The model under review builds one solid part; all positions refer to its coordinate system, in mm. A direction names the side the tool comes from. Round coordinates to 2 decimals unless told otherwise and drop trailing zeros. Order: outer loops, then holes, each group sorted by start corner. A loop starts at its lowest first (then second) coordinate and runs counter-clockwise, first axis right, second up. Notation, with made-up numbers: M -15,-19 L 8,-19 A17 ccw 8,-2 Z; hole C -19,73.5 d5. An arc over 180 degrees is marked long. Use a Markdown table: item, result. Add a question column.
1. To check wall thickness, follow probe 1 along X at (y, z) = (-1, 2.85); probe 2 along Y at (x, z) = (-32, 1.4); probe 3 along Y at (x, z) = (-71.5, 2). State the ranges of each line that lie inside material, in increasing order.
2. For faces 1 (the flat face through (-59.466, 21.267, 1.521)), 2 (the flat face through (-34.34, 12.98, 1.52)), 3 (the flat face through (-17, 0, 1)), 4 (the flat face through (-65.527, -1, 2)), list the 3-axis set-ups (+Z, -Z, +X, -X, +Y, -Y) from which the entire face can be reached by the end or side of a thin tool; tool diameter is ignored.
3. Consider section B-B on x = -8.5. State the section outline as (y, z) points.
4. Consider section A-A on z = 2.55. State the section outline as (x, y) points.
5. Insertion check: P1, Ø1, axis at x = -26, z = 0.5, coming from the +Y side; P2, Ø0.9, axis at x = -10.5, z = 2, coming from the -Y side. Each pin has a flat end and moves straight along its axis. Give the tip position at first contact, or say it passes through.
6. Consider section C-C on y = 13.5. State the section outline as (x, z) points, then the cut area to 3 significant figures.
from build123d import *

# Parameters (mm, degrees)
BOSS_EXTRUDE1_DEPTH = 3
BOSS_EXTRUDE2_DEPTH = 3


with BuildPart() as part:
    # Sketch1 → Boss-Extrude1 (new body)
    with BuildSketch(Plane.XY):
        Polygon((0, 0), (-89, 0), (-80.347524158, 26.629582456), align=None)
    extrude(amount=BOSS_EXTRUDE1_DEPTH)

    # Sketch3 → Boss-Extrude2 (add)
    with BuildSketch(Plane.XY.offset(3)):
        Polygon((-65.527189586, 0), (-65.527189586, -2.933860522), (-33.874345064, -3.087202401), (-33.874345064, 0), align=None)
        Polygon((-59.931116708, 19.862971894), (-58.987312784, 22.710643601), (-33.874345064, 14.38745192), (-34.818148987, 11.539780213), align=None)
    extrude(amount=-BOSS_EXTRUDE2_DEPTH)


solid = part.part
Answer block:
| question | item | result |
|---|---|---|
| 1 | probe 1 | -65.53 to -33.87 |
| 1 | probe 2 | 0 to 10.61 |
| 1 | probe 3 | 0 to 23.7 |
| 2 | face 1 | +Z, -Z, +Y |
| 2 | face 2 | +Z, -Z, +X |
| 2 | face 3 | +Z, -Z, +X, -Y |
| 2 | face 4 | +Z, -Z, -X, -Y |
| 3 | outline | M 0,0 L 2.82,0 L 2.82,3 L 0,3 Z |
| 4 | outline | M -89,0 L -65.53,0 L -65.53,-2.93 L -33.87,-3.09 L -33.87,0 L 0,0 L -34.82,11.54 L -33.87,14.39 L -58.99,22.71 L -59.93,19.86 L -80.35,26.63 Z |
| 5 | P1 | y = 8.78 |
| 5 | P2 | y = 0 |
| 6 | outline | M -84.61,0 L -34.17,0 L -34.17,3 L -84.61,3 Z |
| 6 | area | 151 mm^2 |
